Autodesk Inventor part; units mm, degrees
ref_plane "YZ Plane" through (0, 0, 0) normal (1, 0, 0) x (0, 1, 0)
ref_plane "XZ Plane" through (0, 0, 0) normal (0, 1, 0) x (-1, 0, 0)
ref_plane "XY Plane" through (0, 0, 0) normal (0, 0, 1) x (1, 0, 0)
sketch "Sketch1" plane through (0, 0, 0) normal (0, 1, 0) x (-1, 0, 0)
  line L0 (-23.094, 40) -> (23.094, 40)
  line L1 (23.094, 40) -> (46.188, 0)
  line L2 (46.188, 0) -> (23.094, -40)
  line L3 (23.094, -40) -> (-23.094, -40)
  line L4 (-23.094, -40) -> (-46.188, 0)
  line L5 (-46.188, 0) -> (-23.094, 40)
  line L6 (0, 0) -> (62.8108, 0)
  line L7 (22.6615, -37.7492) -> (1.3, -0.75)
  line L8 (44.023, -0.75) -> (22.6615, -37.7492)
  line L9 (23.094, -40) -> (0, 0) construction
  line L10 (44.023, -0.75) -> (1.3, -0.75)
  line L11 (22.661, 37.75) -> (44.0225, 0.7508)
  line L12 (44.0225, 0.7508) -> (1.2995, 0.7508)
  line L13 (22.661, 37.75) -> (1.2995, 0.7508)
  line L14 (-21.362, 38.5) -> (21.361, 38.5)
  line L15 (21.361, 38.5) -> (-0.0005, 1.5008)
  line L16 (-21.362, 38.5) -> (-0.0005, 1.5008)
  line L17 (-44.023, 0.75) -> (-22.6615, 37.7492)
  line L18 (-22.6615, 37.7492) -> (-1.3, 0.75)
  line L19 (-44.023, 0.75) -> (-1.3, 0.75)
  line L20 (-22.661, -37.75) -> (-44.0225, -0.7508)
  line L21 (-44.0225, -0.7508) -> (-1.2995, -0.7508)
  line L22 (-22.661, -37.75) -> (-1.2995, -0.7508)
  line L23 (21.362, -38.5) -> (-21.361, -38.5)
  line L24 (-21.361, -38.5) -> (0.0005, -1.5008)
  line L25 (21.362, -38.5) -> (0.0005, -1.5008)
  point P0 (0, 0)
  point P1 (0, 0)
  dimension "d6" = 60
  dimension "d7" = 0.75
  dimension "d8" = 1.5
  dimension "d9" = 1.3
  dimension "d10" = 80
  dimension "d13" = 360
extrude "Extrusion1" add sketch "Sketch1" along normal blind 70
sketch "Sketch2" plane through (0, 0, 0) normal (0, -1, 0) x (1, 0, 0)
  line L0 (23.094, 40) -> (46.188, 0)
  line L1 (-23.094, 40) -> (23.094, 40)
  line L2 (-46.188, 0) -> (-23.094, 40)
  line L3 (-23.094, -40) -> (-46.188, 0)
  line L4 (23.094, -40) -> (-23.094, -40)
  line L5 (46.188, 0) -> (23.094, -40)
  line L6 (-21.362, -38.5) -> (21.361, -38.5)
  line L7 (-0.0005, -1.5008) -> (-21.362, -38.5)
  line L8 (21.361, -38.5) -> (-0.0005, -1.5008)
  line L9 (22.661, -37.75) -> (44.0225, -0.7508)
  line L10 (1.2995, -0.7508) -> (22.661, -37.75)
  line L11 (44.0225, -0.7508) -> (1.2995, -0.7508)
  line L12 (44.023, 0.75) -> (22.6615, 37.7492)
  line L13 (1.3, 0.75) -> (44.023, 0.75)
  line L14 (22.6615, 37.7492) -> (1.3, 0.75)
  line L15 (21.362, 38.5) -> (-21.361, 38.5)
  line L16 (0.0005, 1.5008) -> (21.362, 38.5)
  line L17 (-21.361, 38.5) -> (0.0005, 1.5008)
  line L18 (-22.661, 37.75) -> (-44.0225, 0.7508)
  line L19 (-1.2995, 0.7508) -> (-22.661, 37.75)
  line L20 (-44.0225, 0.7508) -> (-1.2995, 0.7508)
  line L21 (-44.023, -0.75) -> (-22.6615, -37.7492)
  line L22 (-1.3, -0.75) -> (-44.023, -0.75)
  line L23 (-22.6615, -37.7492) -> (-1.3, -0.75)
  point P0 (0, 0)
extrude "Extrusion2" add sketch "Sketch2" along normal blind 3 contours L0 L5 L4 L3 L2 L1 | L7 L8 L6 | L10 L11 L9 | L13 L14 L12 | L16 L17 L15 | L19 L20 L18 | L22 L23 L21
sketch "Sketch4" plane through (0, 70, 0) normal (0, 1, 0) x (1, 0, 0)
  line L0 (23.094, -40) -> (46.188, 0)
  line L1 (46.188, 0) -> (23.094, 40)
  line L2 (23.094, 40) -> (-23.094, 40)
  line L3 (-23.094, 40) -> (-46.188, 0)
  line L4 (-46.188, 0) -> (-23.094, -40)
  line L5 (-23.094, -40) -> (23.094, -40)
  line L6 (-21.362, 38.5) -> (21.361, 38.5)
  line L7 (21.361, 38.5) -> (-0.0005, 1.5008)
  line L8 (-0.0005, 1.5008) -> (-21.362, 38.5)
  line L9 (22.661, 37.75) -> (44.0225, 0.7508)
  line L10 (44.0225, 0.7508) -> (1.2995, 0.7508)
  line L11 (1.2995, 0.7508) -> (22.661, 37.75)
  line L12 (44.023, -0.75) -> (22.6615, -37.7492)
  line L13 (22.6615, -37.7492) -> (1.3, -0.75)
  line L14 (1.3, -0.75) -> (44.023, -0.75)
  line L15 (21.362, -38.5) -> (-21.361, -38.5)
  line L16 (-21.361, -38.5) -> (0.0005, -1.5008)
  line L17 (0.0005, -1.5008) -> (21.362, -38.5)
  line L18 (-22.661, -37.75) -> (-44.0225, -0.7508)
  line L19 (-44.0225, -0.7508) -> (-1.2995, -0.7508)
  line L20 (-1.2995, -0.7508) -> (-22.661, -37.75)
  line L21 (-44.023, 0.75) -> (-22.6615, 37.7492)
  line L22 (-22.6615, 37.7492) -> (-1.3, 0.75)
  line L23 (-1.3, 0.75) -> (-44.023, 0.75)
  line L24 (-1.3, 0.75) -> (-44.023, 0.75)
  line L25 (-1.3, 0.75) -> (-0.0005, 1.5008)
  line L26 (-44.023, 0.75) -> (-22.6615, 37.7492)
  line L27 (-21.362, 38.5) -> (21.361, 38.5)
  line L28 (-22.6615, 37.7492) -> (-21.362, 38.5)
extrude "Extrusion3" cut sketch "Sketch4" against normal up to surface (70 mm away) contours L8 L25 L22 L28
pattern_circular "Circular Pattern1" count 2 over 240 about axis through (0, -10, 0) along (0, 1, 0) of "Extrusion3"
chamfer "Chamfer2" distance 7 angle 45 6 edges at (-0.0005, 0, -38.5) (33.3417, 0, -19.2504) (33.3422, 0, 19.2496) (0.0005, 0, 38.5) (-33.3417, 0, 19.2504) (-33.3422, 0, -19.2496)
chamfer "Chamfer1" distance 8 angle 45 6 edges at (34.641, -3, -20) (34.641, -3, 20) (0, -3, 40) (-34.641, -3, 20) (-34.641, -3, -20) (0, -3, -40)
chamfer "Chamfer3" distance 19 angle 45 2 edges at (34.641, 70, -20) (0, 70, -40)
chamfer "Chamfer4" distance 19 angle 45 2 edges at (0, 70, 40) (-34.641, 70, 20)
sketch "Sketch5" plane through (0, 70, 0) normal (0, 1, 0) x (1, 0, 0)
  line L0 (34.0637, -21) -> (32.3316, -21)
  line L1 (34.0637, -21) -> (35.2184, -19)
  line L2 (34.3523, -17.5) -> (35.2184, -19)
  line L3 (34.3523, -17.5) -> (32.3316, -21)
  line L4 (-34.3523, 17.5) -> (-35.2184, 19)
  line L5 (-34.3523, 17.5) -> (-32.3316, 21)
  line L6 (-34.0637, 21) -> (-32.3316, 21)
  line L7 (-34.0637, 21) -> (-35.2184, 19)
  line L8 (-23.094, 40) -> (-34.0637, 21)
  line L9 (-34.0637, 21) -> (-32.3316, 21)
  line L10 (-32.3316, 21) -> (-22.6615, 37.7492)
  line L11 (-22.6615, 37.7492) -> (-21.362, 38.5)
  line L12 (-21.362, 38.5) -> (21.361, 38.5)
  line L13 (21.361, 38.5) -> (11.2574, 21)
  line L14 (11.2574, 21) -> (12.1244, 21)
  line L15 (12.1244, 21) -> (23.094, 40)
  line L16 (23.094, 40) -> (-23.094, 40)
  line L17 (-35.2184, 19) -> (-46.188, 0)
  line L18 (-46.188, 0) -> (-23.094, -40)
  line L19 (-23.094, -40) -> (-12.1244, -21)
  line L20 (-12.1244, -21) -> (-12.5574, -20.25)
  line L21 (-12.5574, -20.25) -> (-22.661, -37.75)
  line L22 (-22.661, -37.75) -> (-44.0225, -0.7508)
  line L23 (-44.0225, -0.7508) -> (-23.8152, -0.7508)
  line L24 (-23.8152, -0.7508) -> (-24.6817, 0.75)
  line L25 (-24.6817, 0.75) -> (-44.023, 0.75)
  line L26 (-44.023, 0.75) -> (-34.3523, 17.5)
  line L27 (-34.3523, 17.5) -> (-35.2184, 19)
  line L28 (12.1244, 21) -> (23.094, 40)
  line L29 (12.1244, 21) -> (12.5574, 20.25)
  line L30 (12.5574, 20.25) -> (22.661, 37.75)
  line L31 (22.661, 37.75) -> (44.0225, 0.7508)
  line L32 (44.023, -0.75) -> (34.3523, -17.5)
  line L33 (34.3523, -17.5) -> (35.2184, -19)
  line L34 (35.2184, -19) -> (46.188, 0)
  line L35 (46.188, 0) -> (23.094, 40)
  line L36 (-23.094, -40) -> (-12.1244, -21)
  line L37 (-23.094, -40) -> (23.094, -40)
  line L38 (23.094, -40) -> (34.0637, -21)
  line L39 (34.0637, -21) -> (32.3316, -21)
  line L40 (32.3316, -21) -> (22.6615, -37.7492)
  line L41 (22.6615, -37.7492) -> (12.9913, -21)
  line L42 (12.9913, -21) -> (11.2583, -21)
  line L43 (11.2583, -21) -> (21.362, -38.5)
  line L44 (21.362, -38.5) -> (-21.361, -38.5)
  line L45 (-21.361, -38.5) -> (-11.2574, -21)
  line L46 (-11.2574, -21) -> (-12.1244, -21)
  line L47 (44.023, -0.75) -> (45.755, -0.75)
  line L48 (22.6615, -37.7492) -> (23.5275, -39.2492)
  line L49 (-22.6615, 37.7492) -> (-23.5275, 39.2492)
  line L50 (-44.023, 0.75) -> (-45.755, 0.75)
  line L51 (0.0005, -1.5008) -> (11.2583, -21)
  line L52 (44.0225, 0.7508) -> (44.023, -0.75)
  point P0 (0, 0)
extrude "Extrusion4" cut sketch "Sketch5" against normal blind 15 contours L38 L48 L40 L0 | L0 L3 L2 L1 | L2 L32 L47 L34 | L17 L4 L26 L50 | L49 L10 L6 L8 | L7 L6 L5 L4
sketch "Sketch6" plane through (0, 70, 0) normal (0, 1, 0) x (1, 0, 0)
  circle A0 centre (-14.6939, 17.2494) radius 16
  ellipse E0 centre (24.2145, -2.943) end of major axis (24.1547, -26.9429) minor radius 17.5
  point P0 (0, 0)
  dimension "d37" = 24
  dimension "d38" = 17.5
  dimension "d36" = 32
properties part number "pen-pot"
Can you work these out from the model? Positions are in its coordinate system, mm. A direction names the side the tool comes from. Give positions to 0.01 mm unless a question says otherwise; leave off trailing zeros. Order: outer loops, then holes, each group sorted by start corner. A loop starts at its lowest first (then second) coordinate and runs counter-clockwise, first axis right, second up. Notation, with made-up numbers: (59.5, 64) - (115.5, 64) arc R20 cw to (115.5, 92) - close; hole circle Ø7 at (27.25, -15). An arc over 180 degrees is marked (long way). Use a Markdown table: item, result. Add a question column.
Q1. If we section it at B-B on x = 6: Write out the boundary of the cut face in (y, z).
Q2. If we section it at C-C on z = -24: Write out the boundary of the cut face in (x, y), plus the area to 3 significant figures.
Q3. On a 3-axis mill with a long thin cutter (end or side, diameter ignored), from which of +Z, -Z, +X, -X, +Y, -Y can I reach the whole of each face in a straight line? I mean faces 5 (the flat face through (-34.803, 29.65, -19.72)), 6 (the flat face through (30.67, 3.55, -16.98)). Say none if no direction works.
Q4. Please list where these lines run through material, in increasing order: line 1 along X through (y, z) = (9.5, 25.5); line 2 along X through (y, z) = (23, 35.5); line 3 along X through (y, z) = (30.5, -34).
Q5. If we mould it in two halves opening along Z, with no side actions, what happens to faces 1 (the flat face through (12.13, 34.51, -19.51)), 2 (the flat face through (0, 28, 40)), 3 (the flat face through (0, 29, -38.5)), 4 (the flat face through (-1, -3, 0))? For each: released by +Z, released by -Z, zero draft, split by the parting line, or undercut.
Q6. If we section it at A-A on y = 10: Write out the boundary of the cut face in (x, z), plus the area to 3 significant figures.
Q7. If we section it at D-D on y = 60: Write out the boundary of the cut face in (x, z), plus the area to 3 significant figures.
Q8. I'm going to push flat-ended pins straight in: pin 1 (6 mm diameter, centred on x = -35.5, z = -18, fed in from +Y); pin 2 (1 mm diameter, centred on x = 36.5, y = 17, fed in from -Z); pin 3 (9 mm diameter, centred on x = -20, z = 16.5, fed in from +Y). Where does each tip first touch, or does it pass through?
Answers follow:
| question | item | result |
|---|---|---|
| 1 | outline | (-3, -32) - (5, -40) - (51, -40) - (52.5, -38.5) - (7, -38.5) - (0, -31.5) - (0, -11.89) - (70, -11.89) - (70, -8.89) - (0, -8.89) - (0, 8.89) - (70, 8.89) - (70, 11.89) - (0, 11.89) - (0, 31.5) - (7, 38.5) - (52.5, 38.5) - (51, 40) - (5, 40) - (-3, 32) - close |
| 2 | outline | (-32.33, 5) - (-23.09, -3) - (23.09, -3) - (32.33, 5) - (32.33, 51) - (30.6, 52.5) - (30.6, 7) - (22.52, 0) - (14.72, 0) - (14.72, 66.25) - (13.86, 67) - (12.99, 67) - (12.99, 0) - (-22.52, 0) - (-30.6, 7) - (-30.6, 55) - (-32.33, 55) - close |
| 2 | area | 477 mm^2 |
| 3 | face 5 | -Z, -X, +Y, -Y |
| 3 | face 6 | +Y |
| 4 | line 1 | x = -31.47 to -29.73, -15.59 to -13.86, 13.86 to 15.59, 29.73 to 31.47 |
| 4 | line 2 | x = -25.69 to -23.96, -21.36 to -19.63, 19.63 to 21.36, 23.96 to 25.69 |
| 4 | line 3 | x = -26.56 to -24.83, 18.76 to 20.5, 24.83 to 26.56 |
| 5 | face 1 | undercut |
| 5 | face 2 | released by +Z |
| 5 | face 3 | undercut |
| 5 | face 4 | zero draft |
| 6 | outline | (-46.19, 0) - (-23.09, -40) - (23.09, -40) - (46.19, 0) - (23.09, 40) - (-23.09, 40) - close; hole (-44.02, -0.75) - (-22.66, -37.75) - (-21.36, -38.5) - (21.36, -38.5) - (0, -1.5) - (-1.3, -0.75) - close; hole (-44.02, 0.75) - (-1.3, 0.75) - (-22.66, 37.75) - close; hole (-21.36, 38.5) - (0, 1.5) - (21.36, 38.5) - close; hole (1.3, -0.75) - (22.66, -37.75) - (44.02, -0.75) - (44.02, 0.75) - (22.66, 37.75) - (1.3, 0.75) - close |
| 6 | area | 672 mm^2 |
| 7 | outline | (-36.23, -0.75) - (-1.3, -0.75) - (0, -1.5) - (17.03, -31) - (17.9, -31) - (18.33, -30.25) - (1.3, -0.75) - (1.3, 0.75) - (18.76, 31) - (17.03, 31) - (0, 1.5) - (-17.03, 31) - (-17.9, 31) - (-18.33, 30.25) - (-1.3, 0.75) - (-35.36, 0.75) - close |
| 7 | area | 212 mm^2 |
| 8 | pin 1 | stops at y = 55 |
| 8 | pin 2 | stops at z = -17.65 |
| 8 | pin 3 | stops at y = 0 |
